The listing builds one solid part. Answer for the finished solid, in the listing's coordinates (mm). A direction names the side the tool comes from. Round coordinates to 2 decimals unless told otherwise and drop trailing zeros. Loops run counter-clockwise (first coordinate to the right, second up) from the corner with the lowest first, then second, coordinate; pieces in that order, holes last. Notation, with made-up numbers: (77, -13.75) -> (116, -13.75) arc R17 ccw to (116, -3.75) -> close; hole circle Ø3 at (-16.75, 21). An arc over 180 degrees is marked (long way). Use a Markdown table: item, result. Add a question column.
Q1. Consider line 1 (Y direction, x = -0.5, z = 1.2); line 2 (Y direction, x = -24, z = 2.3); line 3 (X direction, y = 19, z = 2.9). Determine where each line is inside the solid, lowest interval first.
Q2. Section B-B on x = -11 is taken. Give the vertices of the cut face in (y, z).
Q3. Which of the six approach directions +Z, -Z, +X, -X, +Y, -Y give full straight-line access (tool end or side, diameter ignored) to faces 1 (the flat face through (1.757, 3, 1)), 2 (the flat face through (0, 15, 1)), 3 (the flat face through (-5.021, 62, 1)), 4 (the cylindrical face through (-42.882, 6.594, 1.479)), 5 (the flat face through (-50, 15, 2))?
Q4. Section C-C on y = 13 is taken. Give the vertices of the cut face in (x, z).
Q5. Section D-D on x = -24.5 is taken. Give the vertices of the cut face in (y, z).
Q6. Section A-A on y = 48 is taken. Give the vertices of the cut face in (x, z), then the cut area to 3 significant figures.
Q7. For a pull along X with two mould halves and no side action, classify faces 6 (the flat face through (-48, 60, 1)), 7 (the flat face through (-48.299, 50, 2)), 8 (the cylindrical face through (-42.88, 22.72, 1.48)) as released by +X, released by -X, zero draft, split by the parting line, or undercut.
Q8. Given pin 1 Ø0.9 at (y, z) = (48, 1.5) entering from -X; pin 2 Ø5 at (x, y) = (-8.54, 48) entering from -Z; pin 3 Ø1.5 at (y, z) = (62, 1.5) entering from -X; pin 4 Ø0.9 at (y, z) = (61, 1) entering from +X, each flat-ended and moving along its own axis, determine where each tip first touches the part or whether it passes through.
Autodesk Inventor part; units mm, degrees
ref_plane "YZ Plane" through (0, 0, 0) normal (1, 0, 0) x (0, 1, 0)
ref_plane "XZ Plane" through (0, 0, 0) normal (0, 1, 0) x (-1, 0, 0)
ref_plane "XY Plane" through (0, 0, 0) normal (0, 0, 1) x (1, 0, 0)
sketch "Sketch1" plane through (0, 0, 0) normal (0, 0, 1) x (1, 0, 0)
  line L0 (-16.2709, 3) -> (-16.2709, 0)
  line L1 (-33.7709, 3) -> (-16.2709, 3)
  line L2 (-33.7709, 0) -> (-33.7709, 3)
  line L3 (-33.7709, 0) -> (-48.7992, 0)
  line L4 (-30.0209, 63) -> (-20.0209, 63)
  line L5 (-20.0209, 63) -> (-20.0209, 60)
  line L6 (-30.0209, 60) -> (-30.0209, 63)
  line L7 (-30.0209, 63) -> (-20.0209, 60) construction
  line L8 (-20.0209, 63) -> (-30.0209, 60) construction
  line L9 (-25.4776, 30) -> (-35.4566, 30) construction
  line L10 (-25.0209, 30) -> (-25.0209, 38) construction
  line L11 (-45.0209, 63) -> (-35.0209, 63)
  line L12 (-35.0209, 63) -> (-35.0209, 60)
  line L13 (-45.0209, 60) -> (-45.0209, 63)
  line L14 (-45.0209, 63) -> (-35.0209, 60) construction
  line L15 (-35.0209, 63) -> (-45.0209, 60) construction
  line L16 (-15.0209, 63) -> (-5.0209, 63)
  line L17 (-5.0209, 63) -> (-5.0209, 60)
  line L18 (-15.0209, 60) -> (-15.0209, 63)
  line L19 (-15.0209, 63) -> (-5.0209, 60) construction
  line L20 (-5.0209, 63) -> (-15.0209, 60) construction
  line L21 (-30.0209, 63) -> (-20.0209, 63)
  line L22 (-20.0209, 63) -> (-20.0209, 60)
  line L23 (-30.0209, 60) -> (-30.0209, 63)
  line L24 (-30.0209, 63) -> (-20.0209, 60) construction
  line L25 (-20.0209, 63) -> (-30.0209, 60) construction
  line L26 (-48.7992, 60) -> (-45.0209, 60)
  line L27 (-35.0209, 60) -> (-30.0209, 60)
  line L28 (-20.0209, 60) -> (-15.0209, 60)
  line L29 (-48.7992, 15) -> (-51.799, 15)
  line L30 (-51.799, 15) -> (-51.799, 25)
  line L31 (-51.799, 25) -> (-48.7992, 25)
  line L32 (-48.7992, 35) -> (-51.799, 35)
  line L33 (-51.799, 35) -> (-51.799, 45)
  line L34 (-48.7992, 45) -> (-51.799, 45)
  line L35 (-48.7992, 55) -> (-51.7992, 55)
  line L36 (-48.7992, 55) -> (-45.7992, 55) construction
  line L37 (-51.7992, 55) -> (-51.7992, 60)
  line L38 (-51.7992, 60) -> (-48.7992, 60)
  line L39 (-48.7992, 55) -> (-48.7992, 45)
  line L40 (-48.7992, 35) -> (-48.7992, 25)
  line L41 (-48.7992, 15) -> (-48.7992, 5)
  line L42 (-48.7992, 5) -> (-51.7992, 5)
  line L43 (-51.7992, 5) -> (-51.7992, 0)
  line L44 (-51.7992, 0) -> (-48.7992, 0)
  line L45 (-16.2709, 0) -> (-1.2426, 0)
  line L46 (-1.2426, 60) -> (-5.0209, 60)
  line L47 (-1.2426, 15) -> (1.7572, 15)
  line L48 (1.7572, 15) -> (1.7572, 25)
  line L49 (1.7572, 25) -> (-1.2426, 25)
  line L50 (-1.2426, 35) -> (1.7572, 35)
  line L51 (1.7572, 35) -> (1.7572, 45)
  line L52 (-1.2426, 45) -> (1.7572, 45)
  line L53 (-1.2426, 55) -> (1.7574, 55)
  line L54 (1.7574, 55) -> (1.7574, 60)
  line L55 (1.7574, 60) -> (-1.2426, 60)
  line L56 (-1.2426, 55) -> (-1.2426, 45)
  line L57 (-1.2426, 35) -> (-1.2426, 25)
  line L58 (-1.2426, 15) -> (-1.2426, 5)
  line L59 (-1.2426, 5) -> (1.7574, 5)
  line L60 (1.7574, 5) -> (1.7574, 0)
  line L61 (1.7574, 0) -> (-1.2426, 0)
  circle A0 centre (-44.3959, 23.1933) radius 1.5875
  circle A1 centre (-44.3959, 7.0713) radius 1.5875
  circle A2 centre (-36.7209, 15.1323) radius 8.25
  circle A3 centre (-25.0211, 22.0323) radius 2.95
  circle A4 centre (-25.0211, 8.2323) radius 2.95
  circle A5 centre (-13.3209, 15.1323) radius 8.25
  circle A6 centre (-5.6459, 7.0713) radius 1.5875
  circle A7 centre (-5.6459, 23.1933) radius 1.5875
  circle A8 centre (-41.9566, 29.25) radius 1.5
  circle A9 centre (-41.5, 48) radius 1.5
  line L62 (-5.6459, 7.0713) -> (-44.3959, 23.1933) construction
  line L63 (-44.3959, 23.1933) -> (-5.6459, 23.1933) construction
  line L64 (-5.6459, 23.1933) -> (-44.3959, 7.0713) construction
  point P0 (0, 0)
  point P1 (-25.0209, 61.5)
  point P2 (-40.0209, 61.5)
  point P3 (-10.0209, 61.5)
  point P4 (-25.0209, 61.5)
  point P5 (-48.7992, 30)
  point P6 (-1.2426, 30)
  point P7 (-25.4776, 15.3162)
  point P8 (-25.4776, 15.3162)
  point P9 (-25.4776, 15.3162)
  point P10 (-25.4776, 15.3162)
  point P11 (-25.0209, 3)
  point P12 (-25.0209, 15.1323)
  dimension "d0" = 10
  dimension "d1" = 3
  dimension "d4" = 15
  dimension "d7" = 15
  dimension "d13" = 3
  dimension "d14" = 180
  dimension "d15" = 3
  dimension "d17" = 7.675
  dimension "d18" = 7.675
  dimension "d23" = 2.9998
  dimension "d30" = 11.7002
  dimension "d31" = 11.6998
  dimension "d32" = 7.675
  dimension "d33" = 7.675
  dimension "d34" = 11.6998
  dimension "d35" = 11.7002
  dimension "d45" = 8.061
  dimension "d46" = 8.061
extrude "Extrusion2" add sketch "Sketch1" along normal blind 3
sketch "Sketch2" plane through (0, 0, 3) normal (0, 0, 1) x (1, 0, 0)
  line L0 (-1.2426, 5) -> (-1.2426, 15)
  line L1 (-1.2426, 25) -> (-1.2426, 35)
  line L2 (-1.2426, 45) -> (-1.2426, 55)
  line L3 (-48.7992, 55) -> (-48.7992, 45)
  line L4 (-48.7992, 35) -> (-48.7992, 25)
  line L5 (-48.7992, 15) -> (-48.7992, 5)
  line L6 (-1.2426, 5) -> (-1.7426, 5)
  line L7 (-1.7426, 5) -> (-1.7426, 15)
  line L8 (-1.7426, 15) -> (-1.2426, 15)
  line L9 (-1.2426, 25) -> (-1.7426, 25)
  line L10 (-1.7426, 25) -> (-1.7426, 35)
  line L11 (-1.7426, 35) -> (-1.2426, 35)
  line L12 (-1.2426, 45) -> (-1.7426, 45)
  line L13 (-1.7426, 45) -> (-1.7426, 55)
  line L14 (-1.7426, 55) -> (-1.2426, 55)
  line L15 (-48.7992, 5) -> (-48.2992, 5)
  line L16 (-48.2992, 5) -> (-48.2992, 15)
  line L17 (-48.2992, 15) -> (-48.7992, 15)
  line L18 (-48.7992, 25) -> (-48.2992, 25)
  line L19 (-48.2992, 25) -> (-48.2992, 35)
  line L20 (-48.2992, 35) -> (-48.7992, 35)
  line L21 (-48.7992, 45) -> (-48.2992, 45)
  line L22 (-48.7992, 45) -> (-51.799, 45)
  line L23 (-48.2992, 45) -> (-48.2992, 55)
  line L24 (-48.2992, 55) -> (-48.7992, 55)
  point P0 (0, 0)
  dimension "d24" = 0.5
  dimension "d25" = 0.5
  dimension "d28" = 0.5
  dimension "d29" = 0.5
extrude "Extrusion3" cut sketch "Sketch2" against normal through all
sketch "Sketch3" plane through (0, 0, 3) normal (0, 0, 1) x (1, 0, 0)
  line L0 (-48.2992, 25) -> (-51.799, 25)
  line L1 (-51.799, 25) -> (-51.799, 15)
  line L2 (-51.799, 15) -> (-48.2992, 15)
  line L3 (-48.2992, 15) -> (-48.2992, 5)
  line L4 (-48.2992, 5) -> (-51.7992, 5)
  line L5 (-51.7992, 5) -> (-51.7992, 0)
  line L6 (-51.7992, 0) -> (-33.7709, 0)
  line L7 (-33.7709, 0) -> (-33.7709, 3)
  line L8 (-33.7709, 3) -> (-16.2709, 3)
  line L9 (-16.2709, 3) -> (-16.2709, 0)
  line L10 (-16.2709, 0) -> (1.7574, 0)
  line L11 (1.7574, 0) -> (1.7574, 5)
  line L12 (1.7574, 5) -> (-1.7426, 5)
  line L13 (-1.7426, 5) -> (-1.7426, 15)
  line L14 (-1.7426, 15) -> (1.7572, 15)
  line L15 (1.7572, 15) -> (1.7572, 25)
  line L16 (1.7572, 25) -> (-1.7426, 25)
  line L17 (-1.7426, 25) -> (-1.7426, 35)
  line L18 (-1.7426, 35) -> (1.7572, 35)
  line L19 (1.7572, 35) -> (1.7572, 45)
  line L20 (1.7572, 45) -> (-1.7426, 45)
  line L21 (-1.7426, 45) -> (-1.7426, 55)
  line L22 (-1.7426, 55) -> (1.7574, 55)
  line L23 (1.7574, 55) -> (1.7574, 60)
  line L24 (1.7574, 60) -> (-5.0209, 60)
  line L25 (-5.0209, 60) -> (-5.0209, 63)
  line L26 (-5.0209, 63) -> (-15.0209, 63)
  line L27 (-15.0209, 63) -> (-15.0209, 60)
  line L28 (-15.0209, 60) -> (-20.0209, 60)
  line L29 (-20.0209, 60) -> (-20.0209, 63)
  line L30 (-20.0209, 63) -> (-30.0209, 63)
  line L31 (-30.0209, 63) -> (-30.0209, 60)
  line L32 (-30.0209, 60) -> (-35.0209, 60)
  line L33 (-35.0209, 60) -> (-35.0209, 63)
  line L34 (-35.0209, 63) -> (-45.0209, 63)
  line L35 (-45.0209, 63) -> (-45.0209, 60)
  line L36 (-45.0209, 60) -> (-51.7992, 60)
  line L37 (-51.7992, 60) -> (-51.7992, 55)
  line L38 (-51.7992, 55) -> (-48.2992, 55)
  line L39 (-48.2992, 55) -> (-48.2992, 45)
  line L40 (-48.2992, 45) -> (-51.799, 45)
  line L41 (-51.799, 45) -> (-51.799, 35)
  line L42 (-51.799, 35) -> (-48.2992, 35)
  line L43 (-48.2992, 35) -> (-48.2992, 25)
  circle A0 centre (-13.3209, 15.1323) radius 8.25
  circle A1 centre (-36.7209, 15.1323) radius 8.25
  circle A2 centre (-25.0211, 8.2323) radius 2.95
  circle A3 centre (-25.0211, 22.0323) radius 2.95
  circle A4 centre (-5.6459, 7.0713) radius 1.5875
  circle A5 centre (-5.6459, 23.1933) radius 1.5875
  circle A6 centre (-44.3959, 7.0713) radius 1.5875
  circle A7 centre (-44.3959, 23.1933) radius 1.5875
  circle A8 centre (-41.9566, 29.25) radius 1.5
  circle A9 centre (-41.5, 48) radius 1.5
  line L44 (-25.0211, 33) -> (-25.0211, 49.5)
  circle A10 centre (-8.0855, 29.25) radius 1.5
  circle A11 centre (-8.5422, 48) radius 1.5
  point P0 (0, 0)
extrude "Extrusion4" cut sketch "Sketch3" against normal up to next contours A10 | A11
extrude "Extrusion5" add sketch "Sketch3" against normal blind 3 contours A8 | A9
equation "\"d46\" = d45"
equation "\"d25\" = d24"
equation "\"d28\" = d24"
equation "\"d29\" = d24"
properties part number "srf diag kiri"
Checked values:
| question | item | result |
|---|---|---|
| 1 | line 1 | y = 0 to 5, 15 to 25, 35 to 45, 55 to 60 |
| 1 | line 2 | y = 3 to 5.46, 11 to 19.26, 24.8 to 63 |
| 1 | line 3 | x = -51.8 to -44.01, -29.43 to -20.61, -6.03 to 1.76 |
| 2 | outline | (0, 0) -> (7.22, 0) -> (7.22, 3) -> (0, 3) -> close; (23.05, 0) -> (63, 0) -> (63, 3) -> (23.05, 3) -> close |
| 3 | face 1 | +Z, -Z, +X, +Y, -Y |
| 3 | face 2 | +Z, -Z, +X |
| 3 | face 3 | +Z, -Z, +X, +Y |
| 3 | face 4 | +Z, -Z |
| 3 | face 5 | +Z, -Z, -X |
| 4 | outline | (-48.3, 0) -> (-44.69, 0) -> (-44.69, 3) -> (-48.3, 3) -> close; (-28.75, 0) -> (-21.29, 0) -> (-21.29, 3) -> (-28.75, 3) -> close; (-5.35, 0) -> (-1.74, 0) -> (-1.74, 3) -> (-5.35, 3) -> close |
| 5 | outline | (3, 0) -> (5.33, 0) -> (5.33, 3) -> (3, 3) -> close; (11.14, 0) -> (19.13, 0) -> (19.13, 3) -> (11.14, 3) -> close; (24.94, 0) -> (63, 0) -> (63, 3) -> (24.94, 3) -> close |
| 6 | outline | (-48.3, 0) -> (-10.04, 0) -> (-10.04, 3) -> (-48.3, 3) -> close; (-7.04, 0) -> (-1.74, 0) -> (-1.74, 3) -> (-7.04, 3) -> close |
| 6 | area | 131 mm2 |
| 7 | face 6 | zero draft |
| 7 | face 7 | released by -X |
| 7 | face 8 | undercut |
| 8 | pin 1 | stops at x = -48.3 |
| 8 | pin 2 | stops at z = 0 |
| 8 | pin 3 | stops at x = -45.02 |
| 8 | pin 4 | stops at x = -5.02 |
